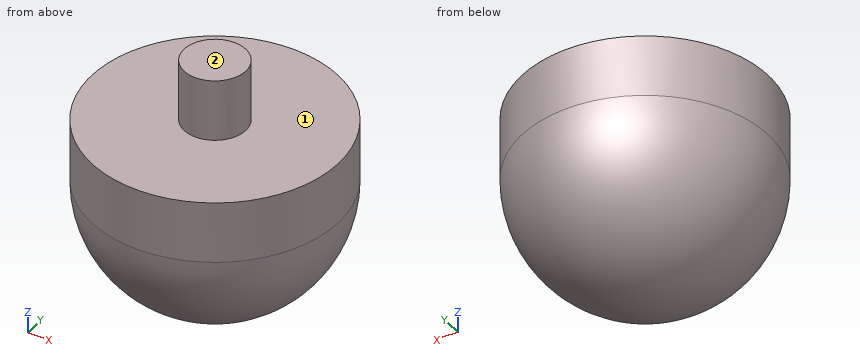
```python
from build123d import *

# Parameters (mm, degrees)
SKETCH1_R           = 20
BOSS_EXTRUDE1_DEPTH = 30
SKETCH2_R           = 5
BOSS_EXTRUDE2_DEPTH = 10
FILLET1_R           = 20


with BuildPart() as part:
    # Sketch1 → Boss-Extrude1 (new body)
    with BuildSketch(Plane.XY):
        Circle(SKETCH1_R)
    extrude(amount=BOSS_EXTRUDE1_DEPTH)

    # Sketch2 → Boss-Extrude2 (add)
    with BuildSketch(Plane.XY.offset(30)):
        Circle(SKETCH2_R)
    extrude(amount=BOSS_EXTRUDE2_DEPTH)

    # Fillet1
    fillet1_edges = [part.edges().sort_by_distance(p)[0] for p in [
        (-20, 0, 0),
    ]]
    fillet(fillet1_edges, radius=FILLET1_R)


solid = part.part
```
The model under review builds one solid part; all positions refer to its coordinate system, in mm. Face numbers are marked on the shaded views. A direction names the side the tool comes from. Give positions to 0.01 mm unless a question says otherwise; leave off trailing zeros. Write each loop counter-clockwise with the first axis right and the second up, starting at its lowest first coordinate (ties: lowest second). Pieces come first, ordered by that corner, then holes.
(1) Consider section C-C, the plane z = 23.5. Give the boundary of the cut face in (x, y), and give its area (3 significant figures).
(2) Tool access review of the marked faces 1 and 2: name each direction out of +Z, -Z, +X, -X, +Y, -Y from which nothing blocks a thin tool from reaching the whole face with its end or side.
(3) For P1, Ø2, axis at x = 1, y = 5, coming from the -Z side; P2, Ø4, axis at x = 10.5, y = -8.5, coming from the -Z side; P3, Ø4, axis at x = 15, z = 26.5, coming from the -Y side, all flat-tipped, find the tip position at first contact; note any pin that passes through.
(4) Consider section D-D, the plane x = 12. Give the boundary of the cut face in (y, z).
(5) To check wall thickness, follow L1, parallel to Y at x = 0, z = 25; L2, parallel to Y at x = 9.5, z = 11.5; L3, parallel to X at y = -2, z = 20. State the ranges of each line that lie inside material, in increasing order.
(6) Consider section A-A, the plane x = 0. Give the boundary of the cut face in (y, z).
Returned:
1. outline: circle Ø40 at (0, 0)
1. area: 1,260 mm2
2. face 1: +Z
2. face 2: +Z, +X, -X, +Y, -Y
3. P1: stops at z = 0.42
3. P2: stops at z = 3.64
3. P3: stops at y = -15.2
4. outline: (-16, 20) arc R16 ccw to (16, 20) - (16, 30) - (-16, 30) - close
5. L1: y = -20 to 20
5. L2: y = -15.41 to 15.41
5. L3: x = -19.9 to 19.9
6. outline: (-20, 20) arc R20 ccw to (20, 20) - (20, 30) - (5, 30) - (5, 40) - (-5, 40) - (-5, 30) - (-20, 30) - close
